from build123d import *

# Parameters (mm, degrees)
F0_W     = 50.8
F0_H     = 50.8
F1_DEPTH = 101.6
F2_R     = 38.1
F3_DEPTH = 304.8
F4_R     = 38.1


with BuildPart() as f1:
    # F0 (on Front) → F1 (new body)
    with BuildSketch(Plane.XZ):
        Rectangle(F0_W, F0_H)
    extrude(amount=F1_DEPTH)

    # F2 (on face) → F3 (join)
    with BuildSketch(Plane.XZ.offset(101.6)):
        Circle(F2_R)
    extrude(amount=F3_DEPTH)

    # F4
    f4_edges = [f1.edges().sort_by_distance(p)[0] for p in [
        (-38.1, -406.4, 0),
    ]]
    fillet(f4_edges, radius=F4_R)


solid = f1.part
Geometry check sheet. Reference: the model listing, model coordinates, mm. A direction names the side the tool comes from. Give positions to 0.01 mm unless a question says otherwise; leave off trailing zeros. Loops run counter-clockwise (first coordinate to the right, second up) from the corner with the lowest first, then second, coordinate; pieces in that order, holes last.
(1) Thickness scan on L1, parallel to Z at x = -1, y = -188; L2, parallel to Z at x = 1, y = -31; L3, parallel to X at y = -312, z = -1.5. Record the ranges inside material, lowest first.
From the geometry:
L1: z = -38.09 to 38.09
L2: z = -25.4 to 25.4
L3: x = -38.07 to 38.07
(2) Section check D-D on y = -375. Record the cut outline in (x, z).
From the geometry:
outline: circle Ø75.01 at (0, 0)
(3) Section check A-A on x = 0. Record the cut outline in (y, z), then the cut area to 3 significant figures.
From the geometry:
outline: (-368.3, -38.1) - (-101.6, -38.1) - (-101.6, -25.4) - (0, -25.4) - (0, 25.4) - (-101.6, 25.4) - (-101.6, 38.1) - (-368.3, 38.1) arc R38.1 ccw to start
area: 27,800 mm2
(4) Set-up check for faces 1 (the flat face through (0, -50, -25.4)), 2 (the flat face through (-25.4, -50, 0)), 3 (the flat face through (0, -50, 25.4)): record each of +Z, -Z, +X, -X, +Y, -Y from which the full face is reachable in a straight line by a thin tool's end or side.
From the geometry:
face 1: -Z, +X, -X, +Y
face 2: +Z, -Z, -X, +Y
face 3: +Z, +X, -X, +Y
(5) Section check B-B on z = -18.5. Record the cut outline in (x, y).
From the geometry:
outline: (-33.31, -368.3) arc R33.31 ccw to (33.31, -368.3) - (33.31, -101.6) - (25.4, -101.6) - (25.4, 0) - (-25.4, 0) - (-25.4, -101.6) - (-33.31, -101.6) - close
(6) Depth check by flat-ended pin: pin 1 Ø2 at (x, z) = (-17.5, -9.5) entering from -Y; pin 2 Ø12 at (y, z) = (-338.5, -20.5) entering from -X; pin 3 Ø3 at (x, y) = (8, -96.5) entering from -Z. Enter the tip coordinate at first touch or a pass-through.
From the geometry:
pin 1: stops at y = -401.37
pin 2: stops at x = -35.23
pin 3: stops at z = -25.4
(7) Section check C-C on y = -263. Record the cut outline in (x, z).
From the geometry:
outline: circle Ø76.2 at (0, 0)
